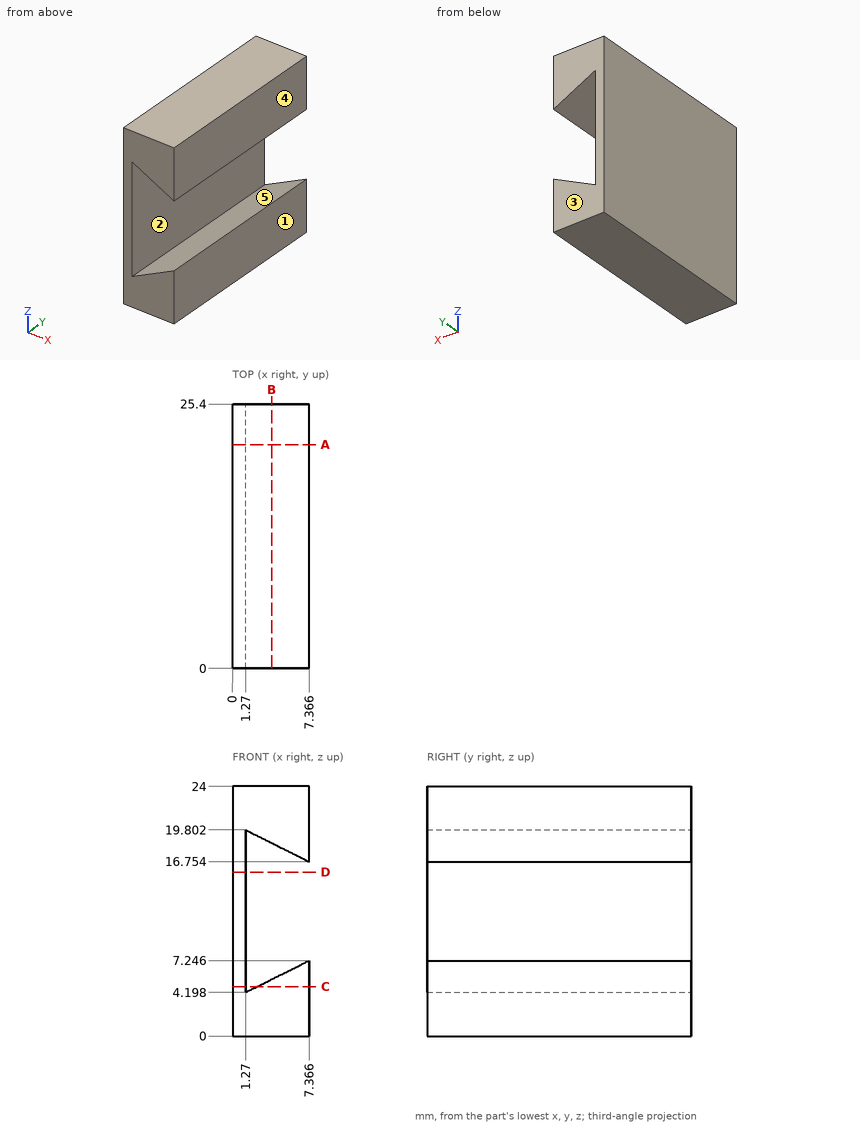
Can you work these out from the drawing? Everything is in mm from the part's minimum corner. A direction names the side the tool comes from. Round coordinates to 2 decimals unless told otherwise and drop trailing zeros. Loops run counter-clockwise (first coordinate to the right, second up) from the corner with the lowest first, then second, coordinate; pieces in that order, holes last. Notation, with made-up numbers: (5, 79.25) -> (37, 79.25) arc R23 cw to (37, 98.25) -> close; hole circle Ø10 at (5.25, 30.25). An arc over 180 degrees is marked (long way). Answer in a Markdown table with one row per item.
Item 1: Suppose I cut it at A-A, the plane y = 21.5. List the corners of the cut face in (x, z) for me.
Answer block:
| item | result |
|---|---|
| outline | (0, 0) -> (7.37, 0) -> (7.37, 7.25) -> (1.27, 4.2) -> (1.27, 19.8) -> (7.37, 16.75) -> (7.37, 24) -> (0, 24) -> close |
Item 2: Suppose I cut it at D-D, the plane z = 15.75. List the corners of the cut face in (x, y) for me, plus the area to 3 significant figures.
Answer block:
| item | result |
|---|---|
| outline | (0, 0) -> (1.27, 0) -> (1.27, 25.4) -> (0, 25.4) -> close |
| area | 32.3 mm² |
Item 3: If I drill on probe 1 along X at (y, z) = (21, 16.5); probe 2 along Z at (x, y) = (6.25, 5); probe 3 along Z at (x, y) = (5.75, 24.25), over which ranges is the centre line in solid material (lowest first)?
Answer block:
| item | result |
|---|---|
| probe 1 | 0 to 1.27 |
| probe 2 | 0 to 6.69, 17.31 to 24 |
| probe 3 | 0 to 6.44, 17.56 to 24 |
Item 4: Suppose I cut it at C-C, the plane z = 4.75. List the corners of the cut face in (x, y) for me.
Answer block:
| item | result |
|---|---|
| outline | (0, 0) -> (1.27, 0) -> (1.27, 25.4) -> (0, 25.4) -> close; (2.37, 0) -> (7.37, 0) -> (7.37, 25.4) -> (2.37, 25.4) -> close |
Item 5: We'd pull the mould along X, two halves only. Please class the marked faces 1, 2 and 3: released by +X, released by -X, zero draft, split by the parting line, or undercut.
Answer block:
| item | result |
|---|---|
| face 1 | released by +X |
| face 2 | undercut |
| face 3 | zero draft |
Item 6: On a 3-axis mill with a long thin cutter (end or side, diameter ignored), from which of +Z, -Z, +X, -X, +Y, -Y can I reach the whole of each face in a straight line? I mean the marked faces 4 and 5. Say none if no direction works.
Answer block:
| item | result |
|---|---|
| face 4 | +Z, -Z, +X, +Y, -Y |
| face 5 | +Y, -Y |
Item 7: Suppose I cut it at B-B, the plane x = 3.75. List the corners of the cut face in (y, z) for me.
Answer block:
| item | result |
|---|---|
| outline | (0, 0) -> (25.4, 0) -> (25.4, 5.44) -> (0, 5.44) -> close; (0, 18.56) -> (25.4, 18.56) -> (25.4, 24) -> (0, 24) -> close |
